Verification items for the finished model (mm, model axes). A direction names the side the tool comes from. Give positions to 0.01 mm unless a question says otherwise; leave off trailing zeros. Loops run counter-clockwise (first coordinate to the right, second up) from the corner with the lowest first, then second, coordinate; pieces in that order, holes last. Notation, with made-up numbers: (-31.75, 40) -> (26.25, 40) arc R25 cw to (26.25, 73) -> close; hole circle Ø1 at (18.25, 1.25). An arc over 180 degrees is marked (long way). Use one line per item in the form item = value. Start each with the question number.
from build123d import *

# Parameters (mm, degrees)
BOSS_EXTRUDE1_DEPTH = 3
FILLET1_R           = 0.2


with BuildPart() as part:
    # Sketch1 → Boss-Extrude1 (new body)
    with BuildSketch(Plane(origin=(0, 0, 0), x_dir=(1, 0, 0), z_dir=(0, 1, 0))):
        with BuildLine():
            Line((-1.5, 0), (-1.5, -3))
            Line((-1.5, -3), (-4, -3))
            ThreePointArc((-4, -3), (-4.353553391, -2.853553391), (-4.5, -2.5))
            Line((-4.5, -2.5), (-4.5, 4.5))
            ThreePointArc((-4.5, 4.5), (-4.353553391, 4.853553391), (-4, 5))
            Line((-4, 5), (3, 5))
            ThreePointArc((3, 5), (3.353553391, 4.853553391), (3.5, 4.5))
            Line((3.5, 4.5), (3.5, 3.243874453))
            ThreePointArc((3.5, 3.243874453), (3.678606195, 2.860852231), (4.086824089, 2.751470576))
            Line((4.086824089, 2.751470576), (10.216965325, 3.832379871))
            ThreePointArc((10.216965325, 3.832379871), (10.590577632, 3.749552017), (10.79619329, 3.426800084))
            Line((10.79619329, 3.426800084), (11.317137823, 0.472376825))
            ThreePointArc((11.317137823, 0.472376825), (11.234309969, 0.098764518), (10.911558035, -0.106851141))
            Line((10.911558035, -0.106851141), (5.495115394, -1.061916118))
            Line((5.495115394, -1.061916118), (3.5, -6))
            Line((3.5, -6), (2, -6))
            ThreePointArc((2, -6), (1.646446609, -5.853553391), (1.5, -5.5))
            Line((1.5, -5.5), (1.5, 0))
            ThreePointArc((1.5, 0), (0, 1.5), (-1.5, 0))
        make_face()
    extrude(amount=BOSS_EXTRUDE1_DEPTH)

    # Fillet1
    fillet1_edges = [part.edges().sort_by_distance(p)[0] for p in [
        (3.353553391, 3, -4.853553391),
        (-0.5, 3, -5),
        (7.151894707, 0, -3.291925224),
        (10.590577632, 0, -3.749552017),
        (11.056665557, 0, -1.949588454),
        (11.234309969, 0, -0.098764518),
        (8.203336715, 0, 0.584383629),
        (-4.353553391, 3, -4.853553391),
        (4.497557697, 0, 3.530958059),
        (2.75, 0, 6),
        (1.646446609, 0, 5.853553391),
        (1.5, 0, 2.75),
        (0, 0, -1.5),
        (-1.5, 0, 1.5),
        (-2.75, 0, 3),
        (-4.353553391, 0, 2.853553391),
        (-4.5, 3, -1),
        (-4.5, 0, -1),
        (-4.353553391, 0, -4.853553391),
        (-0.5, 0, -5),
        (3.353553391, 0, -4.853553391),
        (3.5, 0, -3.871937226),
        (3.678606195, 0, -2.860852231),
        (-4.353553391, 3, 2.853553391),
        (-2.75, 3, 3),
        (-1.5, 1.5, 3),
        (-1.5, 3, 1.5),
        (0, 3, -1.5),
        (1.5, 3, 2.75),
        (1.646446609, 3, 5.853553391),
        (3.678606195, 3, -2.860852231),
        (2.75, 3, 6),
        (4.497557697, 3, 3.530958059),
        (8.203336715, 3, 0.584383629),
        (11.234309969, 3, -0.098764518),
        (11.056665557, 3, -1.949588454),
        (10.590577632, 3, -3.749552017),
        (7.151894707, 3, -3.291925224),
        (3.5, 3, -3.871937226),
    ]]
    fillet(fillet1_edges, radius=FILLET1_R)


solid = part.part
Item 1: Material ranges on line 1 (X direction, y = 0.2, z = -0.5); line 2 (X direction, y = 2.25, z = -4.25); line 3 (Z direction, x = -2.5, y = 0.45), recorded low to high.
Item 2: Tool access check on faces 5 (the flat face through (8.241, 1.482, 0.578)), 6 (the flat face through (-3, 1, 3)), 7 (the flat face through (3.5, 1, -4)), 8 (the cylindrical face through (7.2, 2.94, -3.24)), 9 (the flat face through (1.5, 1, 3)). Record the directions out of +Z, -Z, +X, -X, +Y, -Y that give a thin tool (end or side, any length) a straight path to the whole face; none if there is none.
Item 3: Sectioned sample at B-B, the plane x = 0. Enter the section's corners in (y, z), and give its area (3 significant figures).
Item 4: Draft check along X on faces 1 (the flat face through (3, 1, 6)), 2 (the flat face through (-4.5, 1, -1)), 3 (the flat face through (11.053, 1.482, -1.97)), 4 (the cylindrical face through (0, 1.5, -1.5)). Enter one of: +X half, -X half, draft (parallel to the pull), parting line (faces both ways), or undercut.
Item 5: Gauge pin test, flat ends, axial feed: pin 1 Ø0.8 at (y, z) = (1.5, 3) entering from -X; pin 2 Ø1.3 at (y, z) = (1.5, 0.5) entering from +X; pin 3 Ø1.5 at (x, y) = (6, 1.5) entering from +Z; pin 4 Ø6 at (x, z) = (1.5, 1) entering from -Y. Record the tip position at first contact, or that the pin passes through.
Item 6: Sectioned sample at A-A, the plane y = 2.35. Enter the section's corners in (x, z), and give its area (3 significant figures).
Outcome:
q1.line_1 = -4.5 to -1.41, 1.41 to 11.31
q1.line_2 = -4.5 to 3.5
q1.line_3 = -5 to 3
q2.face_5 = +Z, +X, +Y, -Y
q2.face_6 = +Z, -X, +Y, -Y
q2.face_7 = -Z, +Y, -Y
q2.face_8 = -Z, +Y
q2.face_9 = +Z, +Y, -Y
q3.outline = (0, -4.8) arc R0.2 ccw to (0.2, -5) -> (2.8, -5) arc R0.2 ccw to (3, -4.8) -> (3, -1.7) arc R0.2 ccw to (2.8, -1.5) -> (0.2, -1.5) arc R0.2 ccw to (0, -1.7) -> close
q3.area = 10.5 mm^2
q4.face_1 = draft
q4.face_2 = -X half
q4.face_3 = +X half
q4.face_4 = undercut
q5.pin_1 = -4.49
q5.pin_2 = 11.27
q5.pin_3 = 1.67
q5.pin_4 = 0
q6.outline = (-4.5, -4.5) arc R0.5 ccw to (-4, -5) -> (3, -5) arc R0.5 ccw to (3.5, -4.5) -> (3.5, -3.24) arc R0.5 cw to (4.09, -2.75) -> (10.22, -3.83) arc R0.5 ccw to (10.8, -3.43) -> (11.32, -0.47) arc R0.5 ccw to (10.91, 0.11) -> (5.5, 1.06) -> (3.5, 6) -> (2, 6) arc R0.5 ccw to (1.5, 5.5) -> (1.5, 0) arc R1.5 cw to (-1.5, 0) -> (-1.5, 2.8) arc R0.2 ccw to (-1.7, 3) -> (-4, 3) arc R0.5 ccw to (-4.5, 2.5) -> close
q6.area = 92.5 mm^2
